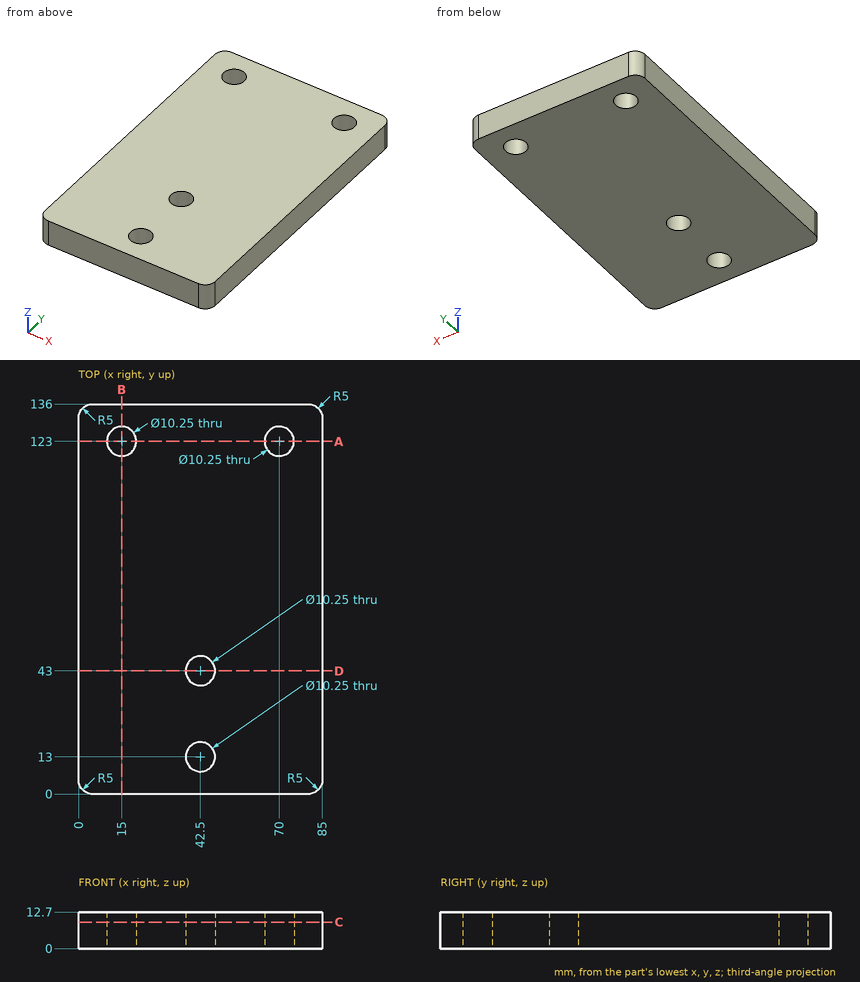
Check sheet for the drawn part. Datum: minimum x, y, z corner. Units: mm. Give positions to 0.01 mm unless a question says otherwise; leave off trailing zeros. Order: outer loops, then holes, each group sorted by start corner. A loop starts at its lowest first (then second) coordinate and runs counter-clockwise, first axis right, second up. Notation, with made-up numbers: (20, 1.5) - (26, 1.5) arc R13 ccw to (26, 16.5) - close; hole circle Ø3 at (2, -16). An arc over 180 degrees is marked (long way). Write item = value, one per line. Start each with the question number.
1) Scan lines: L1, parallel to Y at x = 42.5, z = 3.75 (3 decimals); L2, parallel to Y at x = 45.5, z = 11; L3, parallel to Y at x = 70, z = 7.75 (3 decimals). Record each from-to range of solid material in increasing order.
2) Gauge pin test, flat end, axial feed: pin 1 Ø6 at (x, y) = (42.5, 13) entering from -Z. Record the tip position at first contact, or that the pin passes through.
3) Section check B-B (x = 15). Enter the section's corners in (y, z) (3 decimals).
4) Section check D-D (y = 43). Enter the section's corners in (x, z) (3 decimals), then the cut area to 3 significant figures.
5) Section check C-C (z = 9.25). Enter the section's corners in (x, y) (3 decimals).
6) Section check A-A (y = 123). Enter the section's corners in (x, z) (3 decimals), then the cut area to 3 significant figures.
Geometry check:
q1.L1 = 0 to 7.875, 18.125 to 37.875, 48.125 to 136
q1.L2 = 0 to 8.84, 17.16 to 38.84, 47.16 to 136
q1.L3 = 0 to 117.875, 128.125 to 136
q2.pin_1 = through
q3.outline = (0, 0) - (117.875, 0) - (117.875, 12.7) - (0, 12.7) - close; (128.125, 0) - (136, 0) - (136, 12.7) - (128.125, 12.7) - close
q4.outline = (0, 0) - (37.375, 0) - (37.375, 12.7) - (0, 12.7) - close; (47.625, 0) - (85, 0) - (85, 12.7) - (47.625, 12.7) - close
q4.area = 949 mm2
q5.outline = (0, 5) arc R5 ccw to (5, 0) - (80, 0) arc R5 ccw to (85, 5) - (85, 131) arc R5 ccw to (80, 136) - (5, 136) arc R5 ccw to (0, 131) - close; hole circle Ø10.25 at (15, 123); hole circle Ø10.25 at (42.5, 13); hole circle Ø10.25 at (42.5, 43); hole circle Ø10.25 at (70, 123)
q6.outline = (0, 0) - (9.875, 0) - (9.875, 12.7) - (0, 12.7) - close; (20.125, 0) - (64.875, 0) - (64.875, 12.7) - (20.125, 12.7) - close; (75.125, 0) - (85, 0) - (85, 12.7) - (75.125, 12.7) - close
q6.area = 819 mm2
